```python
from build123d import *

# Parameters (mm, degrees)
SKETCH1_W           = 139.7
SKETCH1_H           = 101.6
BOSS_EXTRUDE1_DEPTH = 5.08
FILLET1_R           = 2.54
SKETCH2_W           = 6.35
SKETCH2_H           = 50.8
BOSS_EXTRUDE2_DEPTH = 139.7
FILLET2_R           = 10.16
SKETCH3_R           = 6.35
CUT_EXTRUDE1_DEPTH  = 119.11


with BuildPart() as part:
    # Sketch1 → Boss-Extrude1 (new body)
    with BuildSketch(Plane(origin=(0, 0, 0), x_dir=(1, 0, 0), z_dir=(0, 1, 0))):
        Rectangle(SKETCH1_W, SKETCH1_H)
        with BuildLine():
            ThreePointArc((-40.325508755, -43.316184338), (-33.204324417, -42.366693093), (-34.153815662, -35.245508755))
            Line((-34.153815662, -35.245508755), (-42.224491245, -29.073815662))
            ThreePointArc((-42.224491245, -29.073815662), (-49.345675583, -30.023306907), (-48.396184338, -37.144491245))
            Line((-48.396184338, -37.144491245), (-40.325508755, -43.316184338))
        make_face(mode=Mode.SUBTRACT)
        with BuildLine():
            ThreePointArc((-48.396184338, 37.144491245), (-49.345675583, 30.023306907), (-42.224491245, 29.073815662))
            Line((-42.224491245, 29.073815662), (-34.153815662, 35.245508755))
            ThreePointArc((-34.153815662, 35.245508755), (-33.204324417, 42.366693093), (-40.325508755, 43.316184338))
            Line((-40.325508755, 43.316184338), (-48.396184338, 37.144491245))
        make_face(mode=Mode.SUBTRACT)
        with BuildLine():
            ThreePointArc((40.325508755, 43.316184338), (33.204324417, 42.366693093), (34.153815662, 35.245508755))
            Line((34.153815662, 35.245508755), (42.224491245, 29.073815662))
            ThreePointArc((42.224491245, 29.073815662), (49.345675583, 30.023306907), (48.396184338, 37.144491245))
            Line((48.396184338, 37.144491245), (40.325508755, 43.316184338))
        make_face(mode=Mode.SUBTRACT)
        with BuildLine():
            Line((48.396184338, -37.144491245), (40.325508755, -43.316184338))
            ThreePointArc((40.325508755, -43.316184338), (33.204324417, -42.366693093), (34.153815662, -35.245508755))
            Line((34.153815662, -35.245508755), (42.224491245, -29.073815662))
            ThreePointArc((42.224491245, -29.073815662), (49.345675583, -30.023306907), (48.396184338, -37.144491245))
        make_face(mode=Mode.SUBTRACT)
    extrude(amount=BOSS_EXTRUDE1_DEPTH)

    # Fillet1
    fillet1_edges = [part.edges().sort_by_distance(p)[0] for p in [
        (69.85, 2.54, -50.8),
        (69.85, 2.54, 50.8),
        (-69.85, 2.54, 50.8),
        (-69.85, 2.54, -50.8),
    ]]
    fillet(fillet1_edges, radius=FILLET1_R)

    # Sketch2 → Boss-Extrude2 (add)
    with BuildSketch(Plane(origin=(0, 5.08, 0), x_dir=(1, 0, 0), z_dir=(0, 1, 0))):
        with Locations((45.085, 0)):
            Rectangle(SKETCH2_W, SKETCH2_H)
        with Locations((-45.085, 0)):
            Rectangle(SKETCH2_W, SKETCH2_H)
    extrude(amount=BOSS_EXTRUDE2_DEPTH)

    # Fillet2
    fillet2_edges = [part.edges().sort_by_distance(p)[0] for p in [
        (-45.085, 144.78, -25.4),
        (-45.085, 144.78, 25.4),
        (45.085, 144.78, -25.4),
        (45.085, 144.78, 25.4),
    ]]
    fillet(fillet2_edges, radius=FILLET2_R)

    # Sketch3 → Cut-Extrude1 (cut, through all)
    with BuildSketch(Plane.ZY.offset(48.26)):
        with Locations((0, 125.73)):
            Circle(SKETCH3_R)
    extrude(amount=-CUT_EXTRUDE1_DEPTH, mode=Mode.SUBTRACT)


solid = part.part
```
Design review of the part built by this model. Coordinates are the model's own, in mm. A direction names the side the tool comes from. Round coordinates to 2 decimals unless told otherwise and drop trailing zeros. Write each loop counter-clockwise with the first axis right and the second up, starting at its lowest first coordinate (ties: lowest second). Pieces come first, ordered by that corner, then holes.
Item 1: We need section C-C on y = 11.5. Write out the cut boundary in (x, z), and give its area (3 significant figures).
Item 2: We need section D-D on x = 3.5. Write out the cut boundary in (y, z).
Item 3: For probe 1 along Z at (x, y) = (45, 125); probe 2 along Y at (x, z) = (-46.25, 0); probe 3 along X at (y, z) = (52, 7), list the stretches that pass through material, from the lowest coordinate up.
Item 4: We need section A-A on y = 125.73. Write out the cut boundary in (x, z), and give its area (3 significant figures).
Item 5: Clearance check with flat-ended pins moving along their axes: pin 1 Ø10 at (y, z) = (112, 7.5) entering from +X; pin 2 Ø1.9 at (x, y) = (45, 86) entering from +Z; pin 3 Ø12 at (x, z) = (-39, 20.5) entering from +Y; pin 4 Ø1.9 at (x, y) = (43.5, 77) entering from -Z. State where each tip first meets the part, or that it passes through.
Item 6: For faces 1 (the flat face through (-38.246, 2.504, -32.116)), 2 (the flat face through (45, 69, -25.4)), 3 (the cylindrical face through (45.129, 141.725, 22.503)), 4 (the flat face through (41.91, 74, 0)), 5 (the flat face through (45, 144.78, 0)), list the 3-axis set-ups (+Z, -Z, +X, -X, +Y, -Y) from which the entire face can be reached by the end or side of a thin tool; tool diameter is ignored.
Item 7: The part is to be moulded in two halves that separate along Z. For faces 6 (the cylindrical face through (45, 132, -1)), 7 (the flat face through (-1, 5.08, -1)), 8 (the cylindrical face through (49.28, 2.5, 29.94)), 9 (the flat face through (-45, 69, 25.4)), say which applies: +Z half, -Z half, draft (parallel to the pull), parting line (faces both ways), or undercut.
Item 8: We need section B-B on z = 0. Write out the cut boundary in (x, y), and give its area (3 significant figures).
Returned:
1. outline: (-48.26, -25.4) - (-41.91, -25.4) - (-41.91, 25.4) - (-48.26, 25.4) - close; (41.91, -25.4) - (48.26, -25.4) - (48.26, 25.4) - (41.91, 25.4) - close
1. area: 645 mm2
2. outline: (0, -50.8) - (5.08, -50.8) - (5.08, 50.8) - (0, 50.8) - close
3. probe 1: z = -25.4 to -6.31, 6.31 to 25.4
3. probe 2: y = 0 to 119.38, 132.08 to 144.78
3. probe 3: x = -48.26 to -41.91, 41.91 to 48.26
4. outline: (-48.26, -25.4) - (-41.91, -25.4) - (-41.91, -6.35) - (-48.26, -6.35) - close; (-48.26, 6.35) - (-41.91, 6.35) - (-41.91, 25.4) - (-48.26, 25.4) - close; (41.91, -25.4) - (48.26, -25.4) - (48.26, -6.35) - (41.91, -6.35) - close; (41.91, 6.35) - (48.26, 6.35) - (48.26, 25.4) - (41.91, 25.4) - close
4. area: 484 mm2
5. pin 1: stops at x = 48.26
5. pin 2: stops at z = 25.4
5. pin 3: stops at y = 144.78
5. pin 4: stops at z = -25.4
6. face 1: +Y, -Y
6. face 2: -Z, +X, -X, +Y
6. face 3: +Z, +X, -X, +Y
6. face 4: +Z, -Z, +Y
6. face 5: +Z, -Z, +X, -X, +Y
7. face 6: undercut
7. face 7: draft
7. face 8: undercut
7. face 9: +Z half
8. outline: (-69.85, 0) - (69.85, 0) - (69.85, 5.08) - (48.26, 5.08) - (48.26, 119.38) - (41.91, 119.38) - (41.91, 5.08) - (-41.91, 5.08) - (-41.91, 119.38) - (-48.26, 119.38) - (-48.26, 5.08) - (-69.85, 5.08) - close; (-48.26, 132.08) - (-41.91, 132.08) - (-41.91, 144.78) - (-48.26, 144.78) - close; (41.91, 132.08) - (48.26, 132.08) - (48.26, 144.78) - (41.91, 144.78) - close
8. area: 2,320 mm2
